Here's how the part is built. I have some questions about the finished solid (model axes, mm). Face numbers are marked on the shaded views. A direction names the side the tool comes from. Coordinates: 2 decimals unless noted, no trailing zeros. Loops run counter-clockwise (first coordinate to the right, second up) from the corner with the lowest first, then second, coordinate; pieces in that order, holes last. Notation, with made-up numbers: M -6.75,-17 L 17.25,-17 A22 cw 17.25,8 Z; hole C 85,-36.5 d8. An arc over 180 degrees is marked long. Use one line per item in the form item = value. Start each with the question number.
(1) Imagine slicing it at B-B, the plane x = 12. Please give me the cut outline in (y, z), and give its area (3 significant figures).
(2) Thinking about a two-plate mould opening in X: for the marked faces 3, 4, 5 and 6, which applies, +X half, -X half, draft (parallel to the pull), parting line (faces both ways), or undercut?
(3) Please list where these lines run through material, in increasing order: L1, parallel to Y at x = 5.25, z = 1.75; L2, parallel to X at y = -4, z = 2; L3, parallel to Y at x = 13.75, z = 2.3.
(4) Imagine slicing it at A-A, the plane y = -0.5. Please give me the cut outline in (x, z), and give its area (3 significant figures).
(5) On a 3-axis mill with a long thin cutter (end or side, diameter ignored), from which of +Z, -Z, +X, -X, +Y, -Y can I reach the whole of each face in a straight line? I mean the marked faces 1 and 2. Say none if no direction works.
(6) Will these pins go through, and if not, where does the flat tip stop? P1, Ø1.1, axis at x = 8, z = 1, coming from the +Y side; P2, Ø3, axis at x = 0, y = -3, coming from the +Z side; P3, Ø1.8, axis at y = -1.5, z = 1, coming from the +X side; P4, Ø1.1, axis at x = 8.5, z = 1, coming from the -Y side.
(7) Imagine slicing it at C-C, the plane z = 0.65. Please give me the cut outline in (x, y).
Autodesk Inventor part; units mm, degrees
ref_plane "YZ Plane" through (0, 0, 0) normal (1, 0, 0) x (0, 1, 0)
ref_plane "XZ Plane" through (0, 0, 0) normal (0, 1, 0) x (-1, 0, 0)
ref_plane "XY Plane" through (0, 0, 0) normal (0, 0, 1) x (1, 0, 0)
sketch "Szkic1" plane through (0, 0, 0) normal (0, 0, 1) x (1, 0, 0)
  line L0 (2.6976, 6.9387) -> (14.6976, 6.9387)
  line L1 (18.6976, 2.9387) -> (18.6976, -4.0613)
  line L2 (14.6976, -8.0613) -> (2.6976, -8.0613)
  line L3 (-1.3024, -4.0613) -> (-1.3024, 2.9387)
  arc A0 (2.6976, 6.9387) -> (-1.3024, 2.9387) centre (2.6976, 2.9387) ccw
  arc A1 (18.6976, 2.9387) -> (14.6976, 6.9387) centre (14.6976, 2.9387) ccw
  arc A2 (14.6976, -8.0613) -> (18.6976, -4.0613) centre (14.6976, -4.0613) ccw
  arc A3 (-1.3024, -4.0613) -> (2.6976, -8.0613) centre (2.6976, -4.0613) ccw
  line L4 (14.6976, 6.4887) -> (2.6976, 6.4887)
  arc A4 (2.6976, 6.4887) -> (-0.8524, 2.9387) centre (2.6976, 2.9387) ccw
  line L5 (-0.8524, 2.9387) -> (-0.8524, -4.0613)
  arc A5 (-0.8524, -4.0613) -> (2.6976, -7.6113) centre (2.6976, -4.0613) ccw
  line L6 (2.6976, -7.6113) -> (14.6976, -7.6113)
  arc A6 (14.6976, -7.6113) -> (18.2476, -4.0613) centre (14.6976, -4.0613) ccw
  line L7 (18.2476, -4.0613) -> (18.2476, 2.9387)
  arc A7 (18.2476, 2.9387) -> (14.6976, 6.4887) centre (14.6976, 2.9387) ccw
  point P0 (0, 0)
  point P1 (18.6976, -8.0613)
  point P2 (18.6976, 6.9387)
  point P3 (-1.3024, -8.0613)
  dimension "d0" = 20
  dimension "d1" = 15
  dimension "d2" = 4
  dimension "d3" = 0.45
extrude "Wyciągnięcie proste1" add sketch "Szkic1" along normal blind 2.2
sketch "Szkic2" plane through (0, 0, 2.2) normal (0, 0, 1) x (1, 0, 0)
  arc A0 (18.2476, 2.9387) -> (14.6976, 6.4887) centre (14.6976, 2.9387) ccw
  line L0 (18.2476, 2.9387) -> (18.2476, -4.0613)
  arc A1 (14.6976, -7.6113) -> (18.2476, -4.0613) centre (14.6976, -4.0613) ccw
  line L1 (14.6976, -7.6113) -> (2.6976, -7.6113)
  arc A2 (-0.8524, -4.0613) -> (2.6976, -7.6113) centre (2.6976, -4.0613) ccw
  line L2 (-0.8524, -4.0613) -> (-0.8524, 2.9387)
  arc A3 (2.6976, 6.4887) -> (-0.8524, 2.9387) centre (2.6976, 2.9387) ccw
  line L3 (2.6976, 6.4887) -> (14.6976, 6.4887)
  line L4 (-1.3024, 2.9387) -> (-1.3024, -4.0613)
  arc A4 (-1.3024, -4.0613) -> (2.6976, -8.0613) centre (2.6976, -4.0613) ccw
  line L5 (2.6976, -8.0613) -> (14.6976, -8.0613)
  arc A5 (14.6976, -8.0613) -> (18.6976, -4.0613) centre (14.6976, -4.0613) ccw
  line L6 (18.6976, -4.0613) -> (18.6976, 2.9387)
  arc A6 (18.6976, 2.9387) -> (14.6976, 6.9387) centre (14.6976, 2.9387) ccw
  line L7 (14.6976, 6.9387) -> (2.6976, 6.9387)
  arc A7 (2.6976, 6.9387) -> (-1.3024, 2.9387) centre (2.6976, 2.9387) ccw
  line L8 (-2.3024, 2.9387) -> (-2.3024, -4.0613)
  arc A8 (-2.3024, -4.0613) -> (2.6976, -9.0613) centre (2.6976, -4.0613) ccw
  line L9 (2.6976, -9.0613) -> (14.6976, -9.0613)
  arc A9 (14.6976, -9.0613) -> (19.6976, -4.0613) centre (14.6976, -4.0613) ccw
  line L10 (19.6976, -4.0613) -> (19.6976, 2.9387)
  arc A10 (19.6976, 2.9387) -> (14.6976, 7.9387) centre (14.6976, 2.9387) ccw
  line L11 (14.6976, 7.9387) -> (2.6976, 7.9387)
  arc A11 (2.6976, 7.9387) -> (-2.3024, 2.9387) centre (2.6976, 2.9387) ccw
  point P0 (0, 0)
  dimension "d6" = 1
extrude "Wyciągnięcie proste2" add sketch "Szkic2" along normal blind 1 contours A7 L7 A6 L6 A5 L5 A4 L4 | A11 L11 A10 L10 A9 L9 A8 L8
sketch "Szkic3" plane through (0, 0, 0) normal (0, 0, -1) x (-1, 0, 0)
  line L0 (2.3024, 2.9387) -> (2.3024, -4.0613)
  arc A0 (2.3024, 2.9387) -> (-2.6976, 7.9387) centre (-2.6976, 2.9387) ccw
  line L1 (-14.6976, 7.9387) -> (-2.6976, 7.9387)
  arc A1 (-14.6976, 7.9387) -> (-19.6976, 2.9387) centre (-14.6976, 2.9387) ccw
  line L2 (-19.6976, -4.0613) -> (-19.6976, 2.9387)
  arc A2 (-19.6976, -4.0613) -> (-14.6976, -9.0613) centre (-14.6976, -4.0613) ccw
  line L3 (-2.6976, -9.0613) -> (-14.6976, -9.0613)
  arc A3 (-2.6976, -9.0613) -> (2.3024, -4.0613) centre (-2.6976, -4.0613) ccw
  arc A4 (1.3024, 2.9387) -> (-2.6976, 6.9387) centre (-2.6976, 2.9387) ccw
  line L4 (1.3024, 2.9387) -> (1.3024, -4.0613)
  arc A5 (-2.6976, -8.0613) -> (1.3024, -4.0613) centre (-2.6976, -4.0613) ccw
  line L5 (-2.6976, -8.0613) -> (-14.6976, -8.0613)
  arc A6 (-18.6976, -4.0613) -> (-14.6976, -8.0613) centre (-14.6976, -4.0613) ccw
  line L6 (-18.6976, -4.0613) -> (-18.6976, 2.9387)
  arc A7 (-14.6976, 6.9387) -> (-18.6976, 2.9387) centre (-14.6976, 2.9387) ccw
  line L7 (-14.6976, 6.9387) -> (-2.6976, 6.9387)
  arc A8 (-14.6976, 6.4887) -> (-18.2476, 2.9387) centre (-14.6976, 2.9387) ccw
  line L8 (-14.6976, 6.4887) -> (-2.6976, 6.4887)
  arc A9 (0.8524, 2.9387) -> (-2.6976, 6.4887) centre (-2.6976, 2.9387) ccw
  line L9 (0.8524, 2.9387) -> (0.8524, -4.0613)
  arc A10 (-2.6976, -7.6113) -> (0.8524, -4.0613) centre (-2.6976, -4.0613) ccw
  line L10 (-2.6976, -7.6113) -> (-14.6976, -7.6113)
  arc A11 (-18.2476, -4.0613) -> (-14.6976, -7.6113) centre (-14.6976, -4.0613) ccw
  line L11 (-18.2476, -4.0613) -> (-18.2476, 2.9387)
  line L12 (1.3024, 2.9387) -> (1.3024, -4.0613)
  arc A12 (1.3024, 2.9387) -> (-2.6976, 6.9387) centre (-2.6976, 2.9387) ccw
  line L13 (-14.6976, 6.9387) -> (-2.6976, 6.9387)
  arc A13 (-14.6976, 6.9387) -> (-18.6976, 2.9387) centre (-14.6976, 2.9387) ccw
  line L14 (-18.6976, -4.0613) -> (-18.6976, 2.9387)
  arc A14 (-18.6976, -4.0613) -> (-14.6976, -8.0613) centre (-14.6976, -4.0613) ccw
  line L15 (-2.6976, -8.0613) -> (-14.6976, -8.0613)
  arc A15 (-2.6976, -8.0613) -> (1.3024, -4.0613) centre (-2.6976, -4.0613) ccw
  point P0 (0, 0)
extrude "Wyciągnięcie proste3" add sketch "Szkic3" along normal blind 1 contours L0 A3 L3 A2 L2 A1 L1 A0 | L4 A5 L5 A6 L6 A7 L7 A4
properties part number "3DP_TPU_Cable_Feed_Through"
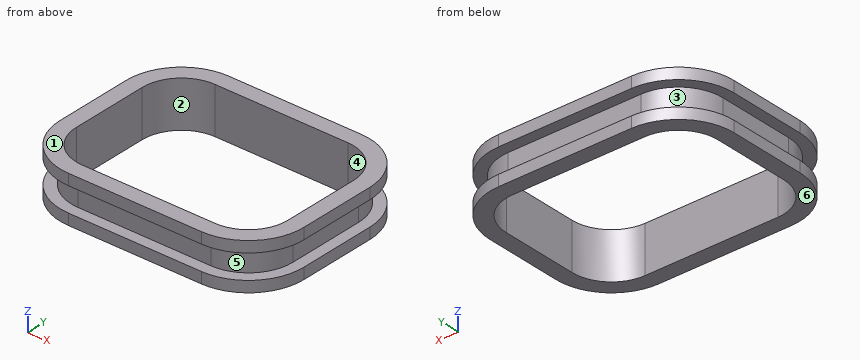
Answer:
q1.outline = M -9.06,-1 L -7.61,-1 L -7.61,3.2 L -9.06,3.2 L -9.06,2.2 L -8.06,2.2 L -8.06,0 L -9.06,0 Z; M 6.49,-1 L 7.94,-1 L 7.94,0 L 6.94,0 L 6.94,2.2 L 7.94,2.2 L 7.94,3.2 L 6.49,3.2 Z
q1.area = 7.78 mm²
q2.face_3 = -X half
q2.face_4 = undercut
q2.face_5 = +X half
q2.face_6 = draft
q3.L1 = -8.06 to -7.61, 6.49 to 6.94
q3.L2 = -1.3 to -0.85, 18.25 to 18.7
q3.L3 = -9.06 to -7.61, 6.49 to 7.94
q4.outline = M -2.3,-1 L -0.85,-1 L -0.85,3.2 L -2.3,3.2 L -2.3,2.2 L -1.3,2.2 L -1.3,0 L -2.3,0 Z; M 18.25,-1 L 19.7,-1 L 19.7,0 L 18.7,0 L 18.7,2.2 L 19.7,2.2 L 19.7,3.2 L 18.25,3.2 Z
q4.area = 7.78 mm²
q5.face_1 = +Z, +X, -X, +Y, -Y
q5.face_2 = +Z, -Z
q6.P1 = 6.94
q6.P2 = 3.2
q6.P3 = 18.7
q6.P4 = -8.06
q7.outline = M -1.3,-4.06 A4 ccw 2.7,-8.06 L 14.7,-8.06 A4 ccw 18.7,-4.06 L 18.7,2.94 A4 ccw 14.7,6.94 L 2.7,6.94 A4 ccw -1.3,2.94 Z; hole M -0.85,-4.06 A3.55 ccw 2.7,-7.61 L 14.7,-7.61 A3.55 ccw 18.25,-4.06 L 18.25,2.94 A3.55 ccw 14.7,6.49 L 2.7,6.49 A3.55 ccw -0.85,2.94 Z
